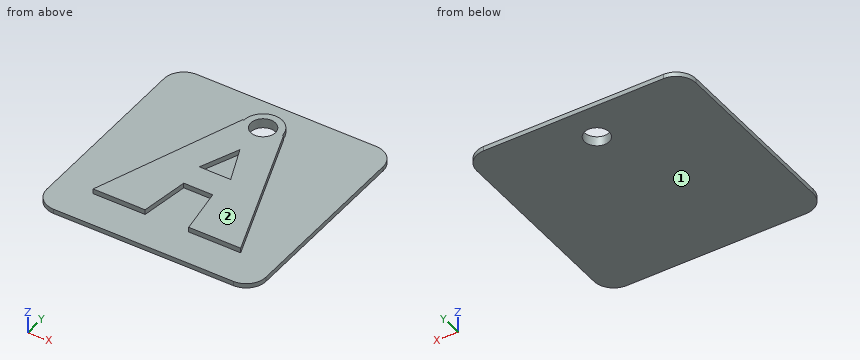
```python
from build123d import *

# Parameters (mm, degrees)
F0_W     = 56.471486
F0_H     = 56.471486
F1_DEPTH = 1.1811
F0_R     = 3.175
F2_DEPTH = 2.4638
F3_R     = 5.08


with BuildPart() as f1:
    # F0 (on Top) → F1 (new body)
    with BuildSketch(Plane.XY):
        Rectangle(F0_W, F0_H)
        with BuildLine():
            Line((4.917035, 19.003581), (5.229957, 19.003581))
            Line((5.229957, 19.003581), (19.003581, -19.003581))
            Line((19.003581, -19.003581), (5.620397, -19.003581))
            Line((5.620397, -19.003581), (3.739397, -6.617126))
            Line((3.739397, -6.617126), (-3.739393, -6.617126))
            Line((-3.739393, -6.617126), (-5.620394, -19.003581))
            Line((-5.620394, -19.003581), (-19.003581, -19.003581))
            Line((-19.003581, -19.003581), (-5.229957, 19.003581))
            Line((-5.229957, 19.003581), (-4.917035, 19.003581))
            ThreePointArc((-4.917035, 19.003581), (0, 23.920617), (4.917035, 19.003581))
        make_face(mode=Mode.SUBTRACT)
        Polygon((0, 9.849461), (-4.047723, 0), (4.047723, 0), align=None)
    extrude(amount=F1_DEPTH)

    # F0 (on Top) → F2 (join)
    with BuildSketch(Plane.XY):
        with BuildLine():
            Line((19.003581, -19.003581), (5.229957, 19.003581))
            Line((5.229957, 19.003581), (4.917035, 19.003581))
            ThreePointArc((4.917035, 19.003581), (0, 23.920617), (-4.917035, 19.003581))
            Line((-4.917035, 19.003581), (-5.229957, 19.003581))
            Line((-5.229957, 19.003581), (-19.003581, -19.003581))
            Line((-19.003581, -19.003581), (-5.620394, -19.003581))
            Line((-5.620394, -19.003581), (-3.739393, -6.617126))
            Line((-3.739393, -6.617126), (3.739397, -6.617126))
            Line((3.739397, -6.617126), (5.620397, -19.003581))
            Line((5.620397, -19.003581), (19.003581, -19.003581))
        make_face()
        Polygon((4.047723, 0), (-4.047723, 0), (0, 9.849461), align=None, mode=Mode.SUBTRACT)
        with Locations((0, 19.003581)):
            Circle(F0_R, mode=Mode.SUBTRACT)
    extrude(amount=F2_DEPTH)

    # F3
    f3_edges = [f1.edges().sort_by_distance(p)[0] for p in [
        (28.235743, 28.235743, 0.59055),
        (-28.235743, 28.235743, 0.59055),
        (-28.235743, -28.235743, 0.59055),
        (28.235743, -28.235743, 0.59055),
    ]]
    fillet(f3_edges, radius=F3_R)


solid = f1.part
```
Input: part model. Units: mm. Frame: model coordinates. Face numbers are marked on the shaded views. Give positions to 0.01 mm unless a question says otherwise; leave off trailing zeros. Order: outer loops, then holes, each group sorted by start corner. A loop starts at its lowest first (then second) coordinate and runs counter-clockwise, first axis right, second up. Notation, with made-up numbers: (71, 71) - (124, 71) arc R25 cw to (124, 87) - close; hole circle Ø10 at (72, 4). An arc over 180 degrees is marked (long way). Put each result on its own line as item: value.
Item 1: Section query D-D, the plane y = 12. Return loops of the section in (x, z), then the cut area to 3 significant figures.
Found:
outline: (-28.24, 0) - (28.24, 0) - (28.24, 1.18) - (7.77, 1.18) - (7.77, 2.46) - (-7.77, 2.46) - (-7.77, 1.18) - (-28.24, 1.18) - close
area: 86.6 mm^2
Item 2: Section query B-B, the plane y = 20. Return loops of the section in (x, z).
Found:
outline: (-28.24, 0) - (-3.01, 0) - (-3.01, 2.46) - (-4.82, 2.46) - (-4.82, 1.18) - (-28.24, 1.18) - close; (3.01, 0) - (28.24, 0) - (28.24, 1.18) - (4.82, 1.18) - (4.82, 2.46) - (3.01, 2.46) - close
Item 3: Contact query for flat-ended pins moving along their axis: pin 1 (1 mm diameter, centred on x = -10, z = 2, fed in from -Y); pin 2 (1 mm diameter, centred on x = 1, y = -19, fed in from +Z). Output: stop coordinate, or through.
Found:
pin 1: stops at y = -19
pin 2: stops at z = 1.18
Item 4: Draft query along Z for the marked faces 1 and 2. Return one class per face: +Z half, -Z half, draft (parallel to the pull), parting line (faces both ways), or undercut.
Found:
face 1: -Z half
face 2: +Z half
Item 5: Ray query, L1, parallel to Y at x = 0, z = 0.85; L2, parallel to Z at x = -3, y = -8.5; L3, parallel to X at y = 4.5, z = 2.2. Return the intervals inside material, ascending. Write a range as from..to.
Found:
L1: y = -28.24..15.83, 22.18..28.24
L2: z = 0..1.18
L3: x = -10.49..-2.2, 2.2..10.49
Item 6: Section query A-A, the plane z = 1.85. Return loops of the section in (x, y) (3 decimals), then the cut area to 3 significant figures.
Found:
outline: (-19.004, -19.004) - (-5.62, -19.004) - (-3.739, -6.617) - (3.739, -6.617) - (5.62, -19.004) - (19.004, -19.004) - (5.23, 19.004) - (4.917, 19.004) arc R4.917 ccw to (-4.917, 19.004) - (-5.23, 19.004) - close; hole (-4.048, 0) - (4.048, 0) - (0, 9.849) - close; hole circle Ø6.35 at (0, 19.004)
area: 772 mm^2
Item 7: Section query C-C, the plane x = 15. Return loops of the section in (y, z), then the cut area to 3 significant figures.
Found:
outline: (-28.24, 0) - (28.24, 0) - (28.24, 1.18) - (-7.96, 1.18) - (-7.96, 2.46) - (-19, 2.46) - (-19, 1.18) - (-28.24, 1.18) - close
area: 80.9 mm^2
